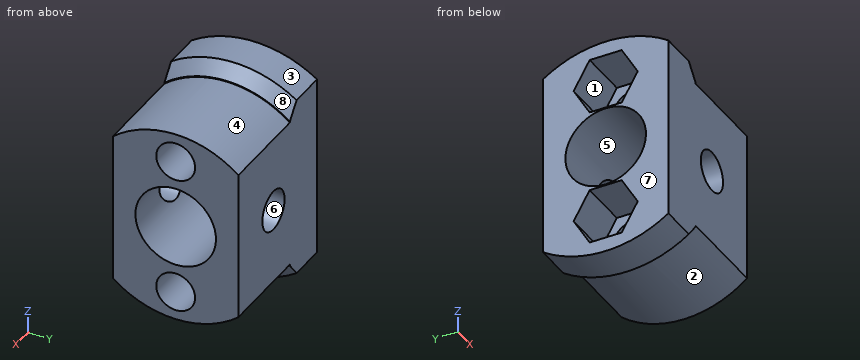
from build123d import *

# Parameters (mm, degrees)
SKETCH1_R                 = 7.9375
SKETCH1_R_2               = 3.2639
SKETCH1_R_3               = 1.575
INNER_SIDE_EXTRUDE_DEPTH  = 2.032
OUTER_START               = -9.525
SKETCH1_3_R               = 7.9375
SKETCH1_3_R_2             = 3.2639
SKETCH1_3_R_3             = 1.575
OUTER_SIDE_EXTRUDE_DEPTH  = 9.525
CLEVIS_PIN_CUT_DEPTH      = 15.721869362
CLEVIS_PIN_CUT_DEPTH_BACK = 15.721869362
SKETCH2_R                 = 1.63195
SKETCH3_R                 = 9
SKETCH3_R_2               = 7.9375
BOSS_EXTRUDE1_DEPTH       = 4
SKETCH4_R                 = 1.575
CUT_EXTRUDE1_DEPTH        = 4
CHAMFER1_SIZE             = 1
CUT_EXTRUDE2_DEPTH        = 16.897346537
CUT_EXTRUDE2_DEPTH_BACK   = 16.897346537
SKETCH5_W                 = 16.51
SKETCH5_H                 = 4.312866645


with BuildPart() as part:
    # Sketch1 → Inner Side Extrude (new body)
    with BuildSketch(Plane(origin=(0, 0, 0), x_dir=(0, 0, -1), z_dir=(1, 0, 0))):
        Circle(SKETCH1_R)
        Circle(SKETCH1_R_2, mode=Mode.SUBTRACT)
        with Locations((-5.588, 0)):
            Circle(SKETCH1_R_3, mode=Mode.SUBTRACT)
        with Locations((5.588, 0)):
            Circle(SKETCH1_R_3, mode=Mode.SUBTRACT)
    extrude(amount=INNER_SIDE_EXTRUDE_DEPTH)

    # Sketch1_3 → Outer Side Extrude (add)
    with BuildSketch(Plane(origin=(0, 0, 0), x_dir=(0, 0, -1), z_dir=(1, 0, 0)).offset(OUTER_START)):
        Circle(SKETCH1_3_R)
        Circle(SKETCH1_3_R_2, mode=Mode.SUBTRACT)
        with Locations((-5.588, 0)):
            Circle(SKETCH1_3_R_3, mode=Mode.SUBTRACT)
        with Locations((5.588, 0)):
            Circle(SKETCH1_3_R_3, mode=Mode.SUBTRACT)
    extrude(amount=OUTER_SIDE_EXTRUDE_DEPTH)

    # Sketch2 → Clevis Pin Cut (cut, two sides: drawn at the far end of the back side and taken through both)
    with BuildSketch(Plane(origin=(0, 0, 0), x_dir=(1, 0, 0), z_dir=(0, 1, 0)).offset(-CLEVIS_PIN_CUT_DEPTH_BACK)):
        with Locations(Location((-3.1242, 0, 0), (0, 0, 270))):
            Circle(SKETCH2_R)
    extrude(amount=CLEVIS_PIN_CUT_DEPTH + CLEVIS_PIN_CUT_DEPTH_BACK, mode=Mode.SUBTRACT)

    # Sketch3 → Boss-Extrude1 (add)
    with BuildSketch(Plane(origin=(-9.525, 0, 0), x_dir=(0, 0, -1), z_dir=(1, 0, 0))):
        Circle(SKETCH3_R)
        Circle(SKETCH3_R_2, mode=Mode.SUBTRACT)
    extrude(amount=BOSS_EXTRUDE1_DEPTH)

    # Sketch4 → Cut-Extrude1 (cut)
    # profile 1 of 2: a face of its own
    with BuildSketch(Plane(origin=(-9.525, 0, 0), x_dir=(0, 0, -1), z_dir=(1, 0, 0))):
        Polygon((-3.338, 1.299038106), (-5.588, 2.598076211), (-7.838, 1.299038106), (-7.838, -1.299038106), (-5.588, -2.598076211), (-3.338, -1.299038106), align=None)
        with Locations(Location((-5.588, 0, 0), (0, 0, 180))):
            Circle(SKETCH4_R, mode=Mode.SUBTRACT)
    # profile 2 of 2: a face of its own
    with BuildSketch(Plane(origin=(-9.525, 0, 0), x_dir=(0, 0, -1), z_dir=(1, 0, 0))):
        Polygon((3.338, 1.299038106), (5.588, 2.598076211), (7.838, 1.299038106), (7.838, -1.299038106), (5.588, -2.598076211), (3.338, -1.299038106), align=None)
        with Locations(Location((5.588, 0, 0), (0, 0, 180))):
            Circle(SKETCH4_R, mode=Mode.SUBTRACT)
    extrude(amount=CUT_EXTRUDE1_DEPTH, mode=Mode.SUBTRACT)

    # Chamfer1
    chamfer1_edges = [part.edges().sort_by_distance(p)[0] for p in [
        (-5.525, 0, 9),
    ]]
    chamfer(chamfer1_edges, length=CHAMFER1_SIZE)

    # Sketch5 → Cut-Extrude2 (cut, two sides: drawn at the far end of the back side and taken through both)
    with BuildSketch(Plane.XY.offset(-CUT_EXTRUDE2_DEPTH_BACK)):
        with Locations((-3.1242, 7.236433322)):
            Rectangle(SKETCH5_W, SKETCH5_H)
        with Locations((-3.1242, -7.236433322)):
            Rectangle(SKETCH5_W, SKETCH5_H)
    extrude(amount=CUT_EXTRUDE2_DEPTH + CUT_EXTRUDE2_DEPTH_BACK, mode=Mode.SUBTRACT)


solid = part.part
Design review of the part built by this model. Coordinates are the model's own, in mm. Face numbers are marked on the shaded views. A direction names the side the tool comes from. Round coordinates to 2 decimals unless told otherwise and drop trailing zeros. Order: outer loops, then holes, each group sorted by start corner. A loop starts at its lowest first (then second) coordinate and runs counter-clockwise, first axis right, second up. Notation, with made-up numbers: M -40,11.5 L -19,11.5 A18 cw -19,17.5 Z; hole C 26.25,4 d4. An arc over 180 degrees is marked long. Answer as CSV lines item,"result". Start each with the question number.
1) Add section A-A (z = 0). Give the boundary of the cut face in (x, y) (3 decimals).
2) Wall thickness on line 1 along X through (y, z) = (3.3, 0) (3 decimals); line 2 along Y through (x, z) = (-6.25, 0); line 3 along Z through (x, y) = (0.75, -1.25): over which ranges is each line inside the solid? List them lowest first. Write a range as [from, to].
3) Tool access review of the marked faces 1, 2, 3, 4 and 5: name each direction out of +Z, -Z, +X, -X, +Y, -Y from which nothing blocks a thin tool from reaching the whole face with its end or side.
4) For pin 1 Ø3.5 at (y, z) = (0, -5.588) entering from -X (3 decimals); pin 2 Ø5 at (x, z) = (-3.12, 0) entering from +Y; pin 3 Ø3 at (y, z) = (0, 5.588) entering from +X, all flat-tipped, find the tip position at first contact; note any pin that passes through.
5) Add section B-B (y = 0). Give the number of separate pieces and of enclosed holes in the cut face, then the cut area to 3 significant figures.
6) The part is to be moulded in two halves that separate along Z. For the marked faces 6, 7 and 8, say which applies: +Z half, -Z half, draft (parallel to the pull), parting line (faces both ways), or undercut.
Resolved:
1,outline,"M -9.525,-5.08 L -4.756,-5.08 L -4.756,-3.264 L -9.525,-3.264 Z; M -9.525,3.264 L -4.756,3.264 L -4.756,5.08 L -9.525,5.08 Z; M -1.492,-5.08 L 2.032,-5.08 L 2.032,-3.264 L -1.492,-3.264 Z; M -1.492,3.264 L 2.032,3.264 L 2.032,5.08 L -1.492,5.08 Z"
2,line 1,"[-9.525, -4.756], [-1.492, 2.032]"
2,line 2,"[-5.08, -3.26], [3.26, 5.08]"
2,line 3,"[-7.84, -6.55], [-4.63, -3.02], [3.02, 4.63], [6.55, 7.84]"
3,face 1,"-X"
3,face 2,"-Z, +X"
3,face 3,"+Z, +X, -X"
3,face 4,"+Z, +X"
3,face 5,"+X, -X"
4,pin 1,"x = -5.525"
4,pin 2,"y = 5.08"
4,pin 3,"through"
5,separate pieces,"4"
5,enclosed holes,"0"
5,area,"31.9 mm^2"
6,face 6,"undercut"
6,face 7,"draft"
6,face 8,"+Z half"
